Could you check a few things on this model? Use its own coordinates, in mm. Face numbers are marked on the shaded views. A direction names the side the tool comes from. Coordinates: 2 decimals unless noted, no trailing zeros. Order: outer loops, then holes, each group sorted by start corner. A loop starts at its lowest first (then second) coordinate and runs counter-clockwise, first axis right, second up. Notation, with made-up numbers: (83, 63.5) - (116, 63.5) arc R22 cw to (116, 80.5) - close; hole circle Ø4 at (81.5, 5.25). An arc over 180 degrees is marked (long way). One line per item, written item: value. Start each with the question number.
from build123d import *

# Parameters (mm, degrees)
BOSS_EXTRU_1_DEPTH           = 19.5
D_GAGEMENT_M3_51_D           = 4.1
D_GAGEMENT_M3_51_DEPTH       = 2
D_GAGEMENT_M2_51_D           = 3.1
D_GAGEMENT_M2_51_ON_FACE_2_D = 3.1


with BuildPart() as part:
    # Esquisse1 → Boss.-Extru.1 (new body)
    with BuildSketch(Plane(origin=(0, 0, 0), x_dir=(0, 0, -1), z_dir=(1, 0, 0))):
        with BuildLine():
            Line((29.85, 15), (29.85, 28.106538385))
            ThreePointArc((29.85, 28.106538385), (25.332375467, 32.237722519), (20.25, 35.650210378))
            Line((20.25, 35.650210378), (20.25, 33.330729065))
            ThreePointArc((20.25, 33.330729065), (24.238194894, 30.553394382), (27.85, 27.301602517))
            Line((27.85, 27.301602517), (27.85, 17))
            Line((27.85, 17), (20.25, 17))
            Line((20.25, 17), (20.25, 15))
            Line((20.25, 15), (29.85, 15))
        make_face()
    extrude(amount=BOSS_EXTRU_1_DEPTH)

    # Dégagement M3.51
    with Locations(Plane(origin=(0, 15, 0), x_dir=(-1, 0, 0), z_dir=(0, -1, 0))):
        with Locations((-15.5, 24.05), (-4, 24.05)):
            Hole(D_GAGEMENT_M3_51_D / 2, depth=D_GAGEMENT_M3_51_DEPTH)

    # Dégagement M2.51 (through all)
    with Locations(Plane(origin=(4, 32.466671627, -25.03827537), x_dir=(0, 0.610689643, 0.79187004), z_dir=(0, 0.79187004, -0.610689643))):
        with Locations((0, 0)):
            Hole(D_GAGEMENT_M2_51_D / 2)

    # Dégagement M2.51 on face 2 (through all)
    with Locations(Plane(origin=(15.5, 32.466671627, -25.03827537), x_dir=(0, 0.610689886, 0.791869852), z_dir=(0, 0.791869852, -0.610689886))):
        with Locations((0, 0)):
            Hole(D_GAGEMENT_M2_51_ON_FACE_2_D / 2)


solid = part.part
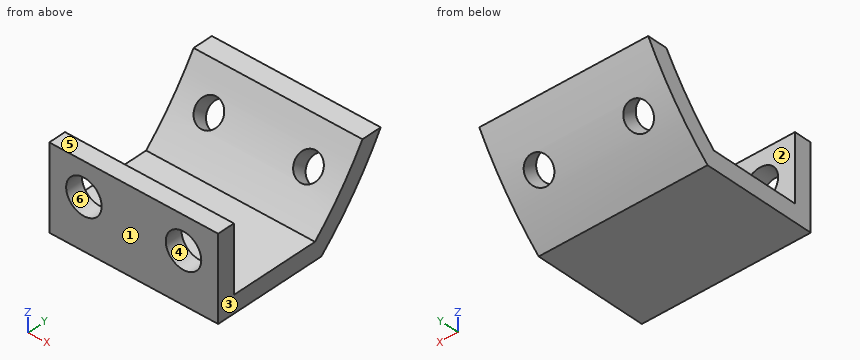
Q1. Which directions (+Z, -Z, +X, -X, +Y, -Y) give clear straight access to the entire face, cutting with the end or side of a thin tool? Please do the marked faces 1 and 2.
Q2. I'm going to push flat-ended pins straight in: pin 1 (5 mm diameter, centred on x = 10.5, y = 21, fed in from +Z); pin 2 (2.5 mm diameter, centred on x = 4, z = -24.05, fed in from -Y); pin 3 (4 mm diameter, centred on y = 25.5, z = -27.5, fed in from +X); pin 4 (4 mm diameter, centred on x = 12, z = -23, fed in from +Y). Where does each tip first touch, or does it pass through?
Q3. I want a section at A-A on x = 6.5. Please give me the cut outline in (y, z), then the cut area to 3 significant figures.
Q4. I want a section at D-D on y = 18.5. Please give me the cut outline in (x, z), then the cut area to 3 significant figures.
Q5. We'd pull the mould along X, two halves only. Please class the marked faces 3, 4, 5 and 6: +X half, -X half, draft (parallel to the pull), parting line (faces both ways), or undercut.
Q6. I want a section at C-C on z = -27.25. Please give me the cut outline in (x, y), then the cut area to 3 significant figures.
Q7. I want a section at B-B on x = 15. Please give me the cut outline in (y, z).
Q8. If I drill on L1, parallel to X at y = 15.75, z = -24.05; L2, parallel to Z at x = 4, y = 15.9; L3, parallel to Z at x = 8.5, y = 23.25, over which ranges is the centre line in solid material (lowest first)?
Values follow:
1. face 1: +Z, -Z, +X, -X, -Y
1. face 2: +Z, +X, -X
2. pin 1: stops at z = -27.85
2. pin 2: stops at y = 29.68
2. pin 3: stops at x = 19.5
2. pin 4: stops at y = 35.21
3. outline: (15, -29.85) - (28.11, -29.85) arc R41 ccw to (35.65, -20.25) - (33.33, -20.25) arc R39 cw to (27.3, -27.85) - (17, -27.85) - (17, -20.25) - (15, -20.25) - close
3. area: 62.6 mm^2
4. outline: (0, -29.85) - (19.5, -29.85) - (19.5, -27.85) - (0, -27.85) - close
4. area: 39.0 mm^2
5. face 3: +X half
5. face 4: undercut
5. face 5: draft
5. face 6: undercut
6. outline: (0, 15) - (19.5, 15) - (19.5, 17) - (0, 17) - close; (0, 27.9) - (19.5, 27.9) - (19.5, 30.63) - (0, 30.63) - close
6. area: 92.3 mm^2
7. outline: (15, -29.85) - (28.11, -29.85) arc R41 ccw to (31.55, -26.18) - (29.97, -24.96) arc R39 cw to (27.3, -27.85) - (17, -27.85) - (17, -26.04) - (15, -26.04) - close; (15, -22.06) - (17, -22.06) - (17, -20.25) - (15, -20.25) - close; (31.76, -22.64) - (33.34, -23.86) arc R41 ccw to (35.65, -20.25) - (33.33, -20.25) arc R39 cw to start
8. L1: x = 0 to 1.95, 6.05 to 13.45, 17.55 to 19.5
8. L2: z = -29.85 to -26.1, -22 to -20.25
8. L3: z = -29.85 to -27.85
